Input: part model. Units: mm. Frame: model coordinates. Face numbers are marked on the shaded views. Round coordinates to 2 decimals unless told otherwise and drop trailing zeros. Loops run counter-clockwise (first coordinate to the right, second up) from the corner with the lowest first, then second, coordinate; pieces in that order, holes last. Notation, with made-up numbers: M 70,43.5 L 122,43.5 A26 cw 122,57.5 Z; hole C 16,83 d4. An arc over 180 degrees is marked long. Return JSON: item names as keys, results as strings. Group by question number.
1) Mould query, pull axis X, two halves, no side actions, for the marked faces 1, 2 and 3. Classes: +X half, -X half, draft (parallel to the pull), parting line (faces both ways), or undercut.
2) Section D-D (x = -4.75). Output: boundary loops of the cut face in (y, z), plus the area to 3 significant figures.
3) Contact query for flat-ended pins moving along their axis: P1, Ø4, axis at x = -2, y = 6.5, coming from the +Z side; P2, Ø4, axis at x = -0.5, y = 5, coming from the -Z side; P3, Ø4, axis at y = 2.5, z = 3.5, coming from the +X side; P4, Ø5, axis at x = 0, z = 0, coming from the -Y side. Output: stop coordinate, or through.
4) Material intervals for line 1 (X direction, y = 5, z = 0); line 2 (Z direction, x = 1.5, y = 3), sorted ascending. Write a range as from..to.
5) Section C-C (y = 1). Output: boundary loops of the cut face in (x, z).
6) Section B-B (z = 0). Output: boundary loops of the cut face in (x, y).
7) Section A-A (x = 0). Output: boundary loops of the cut face in (y, z), plus the area to 3 significant figures.
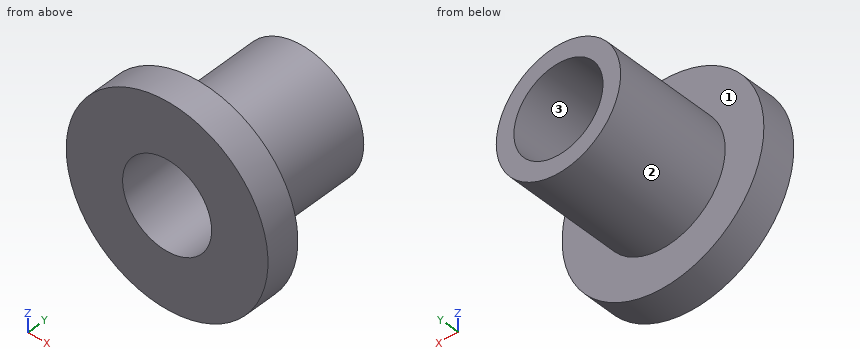
Autodesk Inventor part; units mm, degrees
ref_plane "YZ Plane" through (0, 0, 0) normal (1, 0, 0) x (0, 1, 0)
ref_plane "XZ Plane" through (0, 0, 0) normal (0, 1, 0) x (-1, 0, 0)
ref_plane "XY Plane" through (0, 0, 0) normal (0, 0, 1) x (1, 0, 0)
sketch "Sketch1" plane through (0, 0, 0) normal (0, 1, 0) x (-1, 0, 0)
  circle A0 centre (0, 0) radius 6
  dimension "d0" = 12
extrude "Extrusion1" add sketch "Sketch1" along normal blind 2
sketch "Sketch2" plane through (0, 2, 0) normal (0, 1, 0) x (1, 0, 0)
  circle A0 centre (0, 0) radius 6 construction
  circle A1 centre (0, 0) radius 3.7
  dimension "d3" = 7.4
extrude "Extrusion2" add sketch "Sketch2" along normal blind 7
sketch "Sketch3" plane through (0, 0, 0) normal (0, -1, 0) x (1, 0, 0)
  circle A0 centre (0, 0) radius 6 construction
hole "Hole1" at (0, 0, 0) direction (0, 1, 0) diameter 5.3 end through all
equation "\"d1\" = SPACING"
equation "\"SPACING\" = 2"
properties part number "BearingSpacer"
Returned:
{
 "1": {"face 1": "draft", "face 2": "parting line", "face 3": "undercut"},
 "2": {"outline": "M 0,-3.67 L 2,-3.67 L 2,3.67 L 0,3.67 Z", "area": "14.7 mm^2"},
 "3": {"P1": "stops at z = 3.7", "P2": "stops at z = -3.7", "P3": "stops at x = 5.79", "P4": "passes through"},
 "4": {"line 1": "x = -3.7..-2.65, 2.65..3.7", "line 2": "z = -3.38..-2.18, 2.18..3.38"},
 "5": {"outline": "C 0,0 d12; hole C 0,0 d5.3"},
 "6": {"outline": "M -6,0 L -2.65,0 L -2.65,9 L -3.7,9 L -3.7,2 L -6,2 Z; M 2.65,0 L 6,0 L 6,2 L 3.7,2 L 3.7,9 L 2.65,9 Z"},
 "7": {"outline": "M 0,-6 L 2,-6 L 2,-3.7 L 9,-3.7 L 9,-2.65 L 0,-2.65 Z; M 0,2.65 L 9,2.65 L 9,3.7 L 2,3.7 L 2,6 L 0,6 Z", "area": "28.1 mm^2"}
}
